Work out the finished part from the listing and answer in its coordinate system (mm). Give positions to 0.01 mm unless a question says otherwise; leave off trailing zeros. Loops run counter-clockwise (first coordinate to the right, second up) from the corner with the lowest first, then second, coordinate; pieces in that order, holes last. Notation, with made-up numbers: M 5,8.5 L 10,8.5 A22 cw 10,21.5 Z; hole C 58,22 d5. An arc over 180 degrees is marked long. Use a Markdown table: item, result.
```python
from build123d import *

# Parameters (mm, degrees)
SKETCH_1_R      = 1.85956852
EXTRUDE_1_DEPTH = 3.5
FILLET_1_R      = 1


with BuildPart() as part:
    # 草图1 → 凸台-拉伸1 (new body)
    with BuildSketch(Plane.XY):
        Polygon((-17.433454878, -14.332572831), (-19.600121545, 5.667427169), (19.600121545, 5.667427169), (17.433454878, -14.332572831), align=None)
        with Locations((-5.171924947, -7.35919088)):
            Circle(SKETCH_1_R, mode=Mode.SUBTRACT)
        with Locations(Location((5.171924947, -7.35919088, 0), (0, 0, 180))):
            Circle(SKETCH_1_R, mode=Mode.SUBTRACT)
    extrude(amount=EXTRUDE_1_DEPTH)

    # 圆角1
    fillet_1_edges = [part.edges().sort_by_distance(p)[0] for p in [
        (-17.433454878, -14.332572831, 1.75),
        (-19.600121545, 5.667427169, 1.75),
        (19.600121545, 5.667427169, 1.75),
        (17.433454878, -14.332572831, 1.75),
    ]]
    fillet(fillet_1_edges, radius=FILLET_1_R)


solid = part.part
```
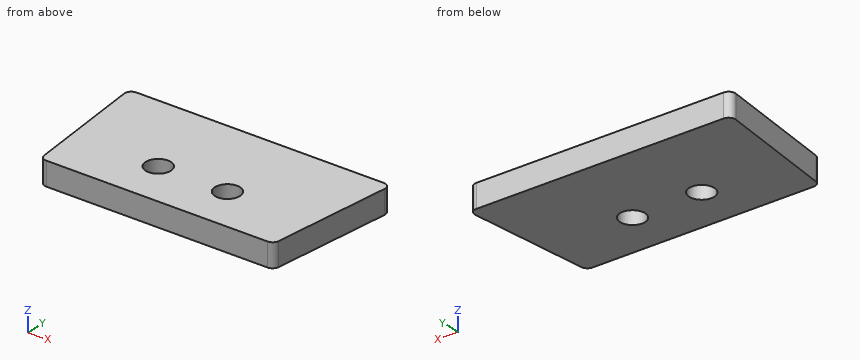
(1) A cutting plane is placed at A-A (x = 5). Write down the section's boundary in (y, z).
Entries:
| item | result |
|---|---|
| outline | M -14.33,0 L -9.21,0 L -9.21,3.5 L -14.33,3.5 Z; M -5.51,0 L 5.67,0 L 5.67,3.5 L -5.51,3.5 Z |
(2) Given P1, Ø5, axis at x = -10, y = 3.5, coming from the -Z side; P2, Ø1.5, axis at y = 0.5, z = 3, coming from the -X side; P3, Ø1.5, axis at y = -7.5, z = 0.5, coming from the +X side, each flat-ended and moving along its own axis, determine where each tip first touches the part or whether it passes through.
Entries:
| item | result |
|---|---|
| P1 | stops at z = 0 |
| P2 | stops at x = -19.12 |
| P3 | stops at x = 18.25 |
(3) A cutting plane is placed at D-D (x = -5.5). Write down the section's boundary in (y, z).
Entries:
| item | result |
|---|---|
| outline | M -14.33,0 L -9.19,0 L -9.19,3.5 L -14.33,3.5 Z; M -5.53,0 L 5.67,0 L 5.67,3.5 L -5.53,3.5 Z |
(4) A cutting plane is placed at B-B (z = 3.05). Write down the section's boundary in (x, y).
Entries:
| item | result |
|---|---|
| outline | M -19.48,4.56 L -17.53,-13.44 A1 ccw -16.54,-14.33 L 16.54,-14.33 A1 ccw 17.53,-13.44 L 19.48,4.56 A1 ccw 18.49,5.67 L -18.49,5.67 A1 ccw Z; hole C -5.17,-7.36 d3.72; hole C 5.17,-7.36 d3.72 |
(5) Consider probe 1 along Y at (x, z) = (5, 3.3); probe 2 along X at (y, z) = (-13.5, 3.3); probe 3 along X at (y, z) = (-9, 2.95). Determine where each line is inside the solid, lowest interval first. Write a range as [from, to].
Entries:
| item | result |
|---|---|
| probe 1 | y = [-14.33, -9.21], [-5.51, 5.67] |
| probe 2 | x = [-17.52, 17.52] |
| probe 3 | x = [-18.01, -6.05], [-4.3, 4.3], [6.05, 18.01] |
(6) A cutting plane is placed at C-C (y = -10.25). Write down the section's boundary in (x, z), and give its area (3 significant figures).
Entries:
| item | result |
|---|---|
| outline | M -17.88,0 L 17.88,0 L 17.88,3.5 L -17.88,3.5 Z |
| area | 125 mm² |
